For this review, take the finished solid that the model builds, in its own axes (mm). A direction names the side the tool comes from. Give positions to 0.01 mm unless a question says otherwise; leave off trailing zeros. Order: outer loops, then holes, each group sorted by start corner. A loop starts at its lowest first (then second) coordinate and runs counter-clockwise, first axis right, second up.
Item 1: Consider section C-C (z = -1.75). Give the boundary of the cut face in (x, y).
Item 2: For P1, Ø1.5, axis at x = 20.5, y = 8, coming from the +Z side; P2, Ø3.5, axis at x = -24, y = -9, coming from the +Z side; P3, Ø5.5, axis at y = 9.5, z = 11, coming from the +X side, all flat-tipped, find the tip position at first contact; note any pin that passes through.
Item 3: Consider section B-B (x = 3). Give the boundary of the cut face in (y, z).
Item 4: For probe 1 along X at (y, z) = (-7.75, 1.75); probe 2 along X at (y, z) = (-1, -1); probe 3 along Z at (x, y) = (-5, -5.25), list the stretches that pass through material, from the lowest coordinate up.
Item 5: Machinability: for faces 4 (the flat face through (-20, -9, -1)), 5 (the flat face through (0, 2, -7.554)), 6 (the flat face through (21, 9, 8)), 7 (the flat face through (23, -6, 3.7)), which of the approach directions +Z, -Z, +X, -X, +Y, -Y give a long, thin tool a straight path to every point of the face, cutting with its end or side? Answer none if there is none.
Item 6: The part is to be moulded in two halves that separate along Z. For faces 1 (the flat face through (0, 13, -9)), 2 (the flat face through (0.378, 2.314, 5.96)), 3 (the flat face through (8.5, 5, -1)), say which applies: released by +Z, released by -Z, zero draft, split by the parting line, or undercut.
Item 7: Consider section D-D (y = -0.25). Give the boundary of the cut face in (x, z).
Item 8: Consider section A-A (y = 11.25). Give the boundary of the cut face in (x, z).
```python
from build123d import *

# Parameters (mm, degrees)
PAD_DEPTH       = 27
SKETCH001_W     = 7
SKETCH001_H     = 26
PAD001_DEPTH    = 16.7
SKETCH002_W     = 11
SKETCH002_H     = 5
POCKET_DEPTH    = 26.001
SKETCH005_W     = 17
SKETCH005_H     = 13.225
POCKET001_DEPTH = 26.001


with BuildPart() as part:
    # Sketch → Pad (new body, symmetric)
    with BuildSketch(Plane.YZ):
        Polygon((8, 13), (-13, -13), (13, -13), (13, 13), align=None)
    extrude(amount=PAD_DEPTH, both=True)

    # Sketch001 (on DatumPlane) → Pad001 (join)
    with BuildSketch(Plane.XY.offset(-13)):
        with Locations((-23.5, 0)):
            Rectangle(SKETCH001_W, SKETCH001_H)
        with Locations((23.5, 0)):
            Rectangle(SKETCH001_W, SKETCH001_H)
    extrude(amount=PAD001_DEPTH)

    # Sketch002 (on DatumPlane) → Pocket (cut, through all)
    with BuildSketch(Plane.XZ.offset(-13)):
        with Locations((-21.5, 10.5)):
            Rectangle(SKETCH002_W, SKETCH002_H)
        with Locations((21.5, 10.5)):
            Rectangle(SKETCH002_W, SKETCH002_H)
    extrude(amount=POCKET_DEPTH, mode=Mode.SUBTRACT)

    # Sketch005 (on DatumPlane) → Pocket001 (cut, through all)
    with BuildSketch(Plane.XZ.offset(-13)):
        with Locations((0, -0.941912)):
            Rectangle(SKETCH005_W, SKETCH005_H)
    extrude(amount=POCKET001_DEPTH, mode=Mode.SUBTRACT)


solid = part.part
```
Resolved:
1. outline: (-27, -13) - (-20, -13) - (-20, -3.91) - (-8.5, -3.91) - (-8.5, 13) - (-27, 13) - close; (8.5, -3.91) - (20, -3.91) - (20, -13) - (27, -13) - (27, 13) - (8.5, 13) - close
2. P1: stops at z = 8
2. P2: stops at z = 3.7
2. P3: stops at x = 16
3. outline: (-13, -13) - (13, -13) - (13, -7.55) - (-8.6, -7.55) - close; (2.08, 5.67) - (13, 5.67) - (13, 13) - (8, 13) - close
4. probe 1: x = -27 to -20, 20 to 27
4. probe 2: x = -27 to -8.5, 8.5 to 27
4. probe 3: z = -13 to -7.55
5. face 4: +Z, -Y
5. face 5: +Y, -Y
5. face 6: +Z, +X, +Y, -Y
5. face 7: +Z, +X, -X, -Y
6. face 1: zero draft
6. face 2: released by +Z
6. face 3: undercut
7. outline: (-27, -13) - (27, -13) - (27, 3.7) - (20, 3.7) - (20, 2.79) - (8.5, 2.79) - (8.5, -7.55) - (-8.5, -7.55) - (-8.5, 2.79) - (-20, 2.79) - (-20, 3.7) - (-27, 3.7) - close
8. outline: (-27, -13) - (27, -13) - (27, 8) - (16, 8) - (16, 13) - (-16, 13) - (-16, 8) - (-27, 8) - close; hole (-8.5, -7.55) - (8.5, -7.55) - (8.5, 5.67) - (-8.5, 5.67) - close
